from build123d import *

# Parameters (mm, degrees)
F0_W     = 187.2611194849
F0_H     = 99.5552539825
F1_DEPTH = 25.4
F2_SIZE  = 25.39999


# Not quite as in the source:
# - a fillet or chamfer is up to 0.001 mm smaller than in the source, because OpenCascade refuses the exact size


with BuildPart() as f1:
    # F0 (on Top) → F1 (new body)
    with BuildSketch(Plane.XY):
        Rectangle(F0_W, F0_H)
    extrude(amount=F1_DEPTH)

    # F2 (size 25.4 in the source; OpenCascade refuses exactly that, so slightly less here)
    f2_edges = [f1.edges().sort_by_distance(p)[0] for p in [
        (-93.63056, 0, 0),
        (93.63056, 0, 0),
    ]]
    chamfer(f2_edges, length=F2_SIZE)


solid = f1.part
Could you check a few things on this model? Use its own coordinates, in mm. Round coordinates to 2 decimals unless told otherwise and drop trailing zeros. Write each loop counter-clockwise with the first axis right and the second up, starting at its lowest first coordinate (ties: lowest second). Pieces come first, ordered by that corner, then holes. Notation, with made-up numbers: (-39, 88.5) -> (-11, 88.5) arc R25 cw to (-11, 108.5) -> close; hole circle Ø1 at (-3.75, 68.25). An arc over 180 degrees is marked (long way). Use a Markdown table: item, result.
1. For pin 1 Ø1 at (y, z) = (-6.5, 5) entering from -X; pin 2 Ø6 at (y, z) = (-21.5, 13) entering from -X, each with a flat end and sliding along its axis, tell me the tip position at first contact or that it passes through.
Answer key:
| item | result |
|---|---|
| pin 1 | stops at x = -73.73 |
| pin 2 | stops at x = -84.23 |
2. Please list where these lines run through material, in increasing order: probe 1 along Z at (x, y) = (-70.5, -25.5); probe 2 along X at (y, z) = (-1.5, 20.25); probe 3 along Z at (x, y) = (-75, -32).
Answer key:
| item | result |
|---|---|
| probe 1 | z = 2.27 to 25.4 |
| probe 2 | x = -88.48 to 88.48 |
| probe 3 | z = 6.77 to 25.4 |
3. If we section it at C-C (x = 82): List the corners of the cut face in (y, z) for me.
Answer key:
| item | result |
|---|---|
| outline | (-49.78, 13.77) -> (49.78, 13.77) -> (49.78, 25.4) -> (-49.78, 25.4) -> close |
